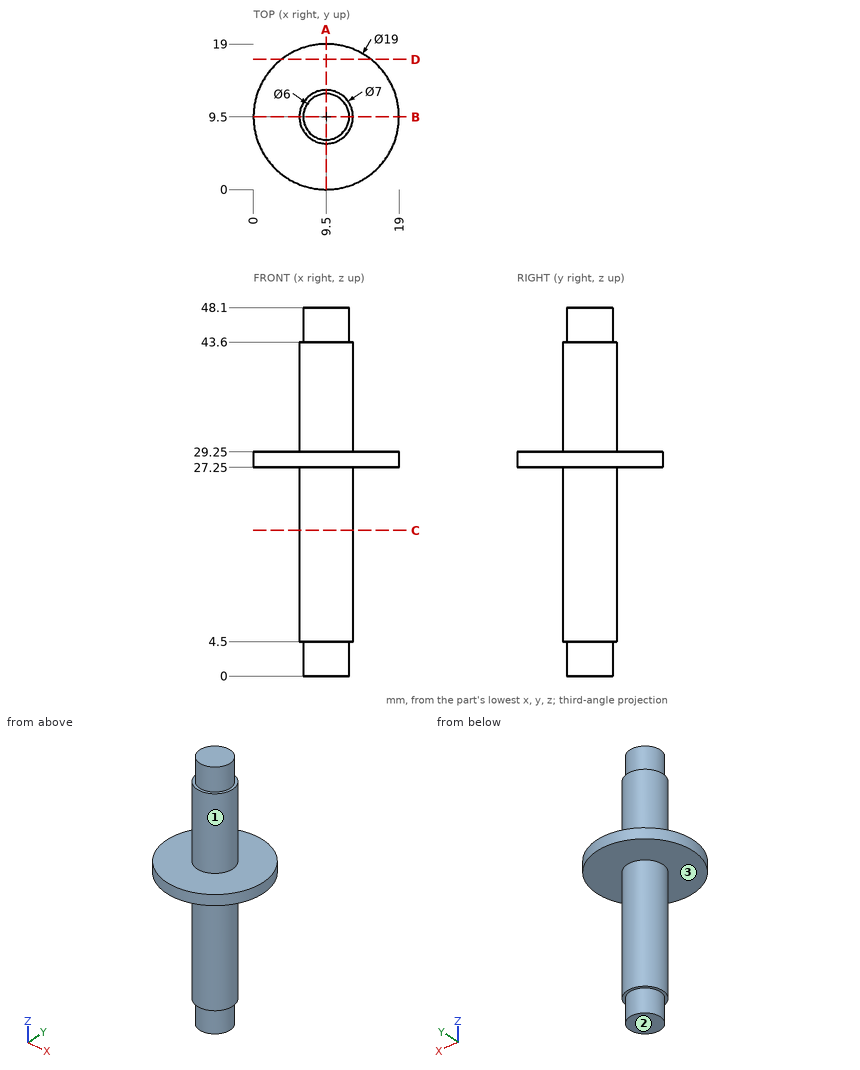
Check sheet for the drawn part. Datum: minimum x, y, z corner. Units: mm. A direction names the side the tool comes from. Coordinates: 2 decimals unless noted, no trailing zeros. Loops run counter-clockwise (first coordinate to the right, second up) from the corner with the lowest first, then second, coordinate; pieces in that order, holes last. Notation, with made-up numbers: (83.25, 69.5) -> (98.25, 69.5) arc R5 cw to (98.25, 74.5) -> close; hole circle Ø8 at (63, 87.25). An arc over 180 degrees is marked (long way). Answer as a JSON object with one key per item and string values. Group by question number.
Item 1: Depth check by flat-ended pin: pin 1 (1.5 mm diameter, centred on x = 14.5, y = 2.5, fed in from -Z); pin 2 (2 mm diameter, centred on y = 7.5, z = 18, fed in from -X); pin 3 (1 mm diameter, centred on y = 13, z = 32.5, fed in from +X); pin 4 (3 mm diameter, centred on x = 3, z = 21, fed in from +Y). Enter the tip coordinate at first touch or a pass-through.
Item 2: Sectioned sample at A-A on x = 9.5. Record the boundary of the cut face in (y, z).
Item 3: Sectioned sample at D-D on y = 17. Record the boundary of the cut face in (x, z).
Item 4: Tool access check on the marked faces 1, 2 and 3. Record the directions out of +Z, -Z, +X, -X, +Y, -Y that give a thin tool (end or side, any length) a straight path to the whole face; none if there is none.
Item 5: Sectioned sample at C-C on z = 19. Record the boundary of the cut face in (x, y), plus the area to 3 significant figures.
Item 6: Scan lines: probe 1 along Z at (x, y) = (14.5, 16); probe 2 along X at (y, z) = (9.75, 22); probe 3 along X at (y, z) = (12.25, 20). Record each from-to range of solid material in increasing order.
Evaluation:
{
 "1": {"pin 1": "stops at z = 27.25", "pin 2": "stops at x = 6.15", "pin 3": "stops at x = 11.3", "pin 4": "passes through"},
 "2": {"outline": "(0, 27.25) -> (6, 27.25) -> (6, 4.5) -> (6.5, 4.5) -> (6.5, 0) -> (12.5, 0) -> (12.5, 4.5) -> (13, 4.5) -> (13, 27.25) -> (19, 27.25) -> (19, 29.25) -> (13, 29.25) -> (13, 43.6) -> (12.5, 43.6) -> (12.5, 48.1) -> (6.5, 48.1) -> (6.5, 43.6) -> (6, 43.6) -> (6, 29.25) -> (0, 29.25) -> close"},
 "3": {"outline": "(3.67, 27.25) -> (15.33, 27.25) -> (15.33, 29.25) -> (3.67, 29.25) -> close"},
 "4": {"face 1": "+Z", "face 2": "-Z, +X, -X, +Y, -Y", "face 3": "-Z"},
 "5": {"outline": "circle Ø7 at (9.5, 9.5)", "area": "38.5 mm²"},
 "6": {"probe 1": "z = 27.25 to 29.25", "probe 2": "x = 6.01 to 12.99", "probe 3": "x = 7.33 to 11.67"}
}
